from build123d import *

# Parameters (mm, degrees)
CUT_EXTRUDE_1_DEPTH         = 299.559693571
CUT_EXTRUDE_1_DEPTH_BACK    = 299.559693571
SKETCH_2_W                  = 19
SKETCH_2_H                  = 9.5
SKETCH_3_R                  = 55
EXTRUDE_1_DEPTH             = 2
SKETCH_4_W                  = 19
SKETCH_4_H                  = 9.5
CUT_EXTRUDE_2_DEPTH         = 2
HOLE_WIZARD_M41_D           = 4.5
PATTERN_CIRCULAR_1_COUNT    = 4
HOLE_WIZARD_M42_D           = 4.5
HOLE_WIZARD_M42_DEPTH       = 10
HOLE_WIZARD_M42_CSINK_D     = 4.55
HOLE_WIZARD_M42_CSINK_ANGLE = 90
HOLE_WIZARD_M42_TIP         = 1.351936393


with BuildPart() as part:
    # Sketch 1 → Revolve 1 (revolve)
    with BuildSketch(Plane(origin=(0, 0, 0), x_dir=(1, 0, 0), z_dir=(0, 1, 0)), mode=Mode.PRIVATE) as revolve_1_sk:
        Polygon((0, 0), (200, 0), (200, -27.777777778), (210, -30.625), (210, 10), (0, 10), align=None)
    revolve(revolve_1_sk.sketch.rotate(Axis((0, 0, -10), (0, 0, 1)), 180), axis=Axis((0, 0, -10), (0, 0, 1)))

    # Sketch 2 → Cut-Extrude 1 (cut, two sides: drawn at the far end of the back side and taken through both)
    with BuildSketch(Plane.XY.offset(-CUT_EXTRUDE_1_DEPTH_BACK)):
        Rectangle(SKETCH_2_W, SKETCH_2_H)
    extrude(amount=CUT_EXTRUDE_1_DEPTH + CUT_EXTRUDE_1_DEPTH_BACK, mode=Mode.SUBTRACT)

    # Sketch 3 → Extrude 1 (add)
    with BuildSketch(Plane.XY):
        with Locations(Location((0, 0, 0), (0, 0, 180))):
            Circle(SKETCH_3_R)
    extrude(amount=EXTRUDE_1_DEPTH)

    # Sketch 4 → Cut-Extrude 2 (cut)
    with BuildSketch(Plane.XY.offset(2)):
        Rectangle(SKETCH_4_W, SKETCH_4_H)
    extrude(amount=-CUT_EXTRUDE_2_DEPTH, mode=Mode.SUBTRACT)

    # Hole Wizard M41 (through all)
    with Locations(Plane(origin=(0, 45, 2), x_dir=(1, 0, 0), z_dir=(0, 0, 1))):
        with Locations((0, 0)):
            hole_wizard_m41 = Hole(HOLE_WIZARD_M41_D / 2)

    # Pattern Circular 1: Hole Wizard M41 ×4 about axis
    pattern_circular_1_axis = Axis((0, 0, 0), (0, 0, 1))
    for i in range(1, PATTERN_CIRCULAR_1_COUNT):
        add(hole_wizard_m41.rotate(pattern_circular_1_axis, i * 360 / PATTERN_CIRCULAR_1_COUNT), mode=Mode.SUBTRACT)

    # Hole Wizard M42
    with Locations(Plane(origin=(-14.5, 15, -10), x_dir=(-1, 0, 0), z_dir=(0, 0, -1))):
        with Locations((0, 0), (-29, 0), (-29, -30), (0, -30)):
            CounterSinkHole(HOLE_WIZARD_M42_D / 2, HOLE_WIZARD_M42_CSINK_D / 2, depth=HOLE_WIZARD_M42_DEPTH, counter_sink_angle=HOLE_WIZARD_M42_CSINK_ANGLE)
            with Locations((0, 0, -(HOLE_WIZARD_M42_DEPTH + HOLE_WIZARD_M42_TIP / 2))):  # 118° drill point
                Cone(0, HOLE_WIZARD_M42_D / 2, HOLE_WIZARD_M42_TIP, mode=Mode.SUBTRACT)


solid = part.part
Verification items for the finished model (mm, model axes). A direction names the side the tool comes from. Give positions to 0.01 mm unless a question says otherwise; leave off trailing zeros. Write each loop counter-clockwise with the first axis right and the second up, starting at its lowest first coordinate (ties: lowest second). Pieces come first, ordered by that corner, then holes. Notation, with made-up numbers: (-8, -1.5) - (49, -1.5) arc R26 cw to (49, 20.5) - close; hole circle Ø2 at (-8.5, 41.25). An arc over 180 degrees is marked (long way). Answer as CSV lines item,"result". Start each with the question number.
1. Thickness scan on line 1 (Y direction, x = 0, z = -3.75); line 2 (Y direction, x = -14.5, z = -6); line 3 (X direction, y = 15, z = -5). Record the ranges inside material, lowest first.
2. Set-up check for faces 4 (the face through (-9.5, 0, -4)), 5 (the face through (1, 11, 2)): record each of +Z, -Z, +X, -X, +Y, -Y from which the full face is reachable in a straight line by a thin tool's end or side.
3. Sectioned sample at A-A (z = 7). Record the boundary of the cut face in (x, y), then the cut area to 3 significant figures.
4. Depth check by flat-ended pin: pin 1 (4 mm diameter, centred on x = 45, z = 11.5, fed in from -Y); pin 2 (2.5 mm diameter, centred on x = -45, y = 0, fed in from -Z); pin 3 (5 mm diameter, centred on x = -14.5, y = -15, fed in from +Z); pin 4 (10 mm diameter, centred on x = -134.5, z = 1, fed in from -Y). Enter the tip coordinate at first touch or a pass-through.
5. Draft check along X on faces 1 (the face through (9.5, 0, -4)), 2 (the face through (3, 44, -10)), 3 (the face through (-200.3, -63.08, 10.03)). Enter one of: pulls with the +X half, pulls with the -X half, needs draft (parallel to the pull), parting line crosses it, or undercut.
Derived:
1,line 1,"-210 to -47.25, -42.75 to -4.75, 4.75 to 42.75, 47.25 to 210"
1,line 2,"-209.5 to -17.25, -12.75 to 12.75, 17.25 to 209.5"
1,line 3,"-209.46 to -16.75, -12.25 to 12.25, 16.75 to 209.46"
2,face 4,"+Z, -Z"
2,face 5,"+Z"
3,outline,"circle Ø420 at (0, 0); hole circle Ø400 at (0, 0)"
3,area,"12,900 mm²"
4,pin 1,"y = -205.55"
4,pin 2,"through"
4,pin 3,"z = 2"
4,pin 4,"y = -165.32"
5,face 1,"undercut"
5,face 2,"needs draft"
5,face 3,"parting line crosses it"
